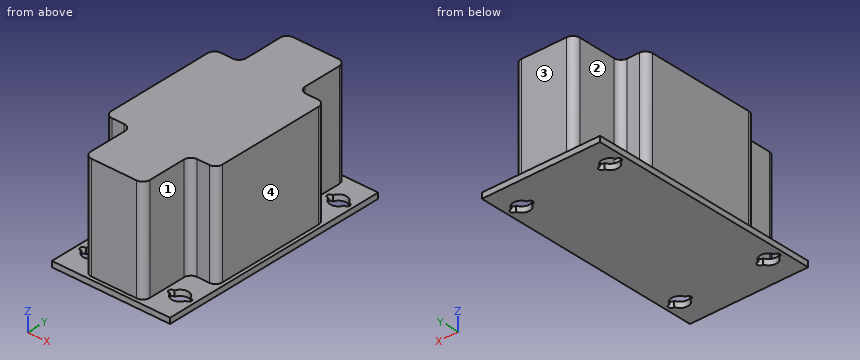
Autodesk Inventor part; units mm, degrees
ref_plane "YZ Plane" through (0, 0, 0) normal (1, 0, 0) x (0, 1, 0)
ref_plane "XZ Plane" through (0, 0, 0) normal (0, 1, 0) x (-1, 0, 0)
ref_plane "XY Plane" through (0, 0, 0) normal (0, 0, 1) x (1, 0, 0)
sketch "Sketch1" plane through (0, 0, 0) normal (0, 0, 1) x (1, 0, 0)
  line L0 (17, 33.5) -> (-17, 33.5)
  line L1 (-17, 33.5) -> (-17, -33.5)
  line L2 (-17, -33.5) -> (17, -33.5)
  line L3 (17, -33.5) -> (17, 33.5)
  line L4 (17, 33.5) -> (-17, -33.5) construction
  line L5 (-17, 33.5) -> (17, -33.5) construction
  line L6 (-12.75, 25.5) -> (12.75, 25.5) construction
  line L7 (12.75, 25.5) -> (12.75, -25.5) construction
  line L8 (12.75, -25.5) -> (-12.75, -25.5) construction
  line L9 (-12.75, -25.5) -> (-12.75, 25.5) construction
  line L10 (-12.75, 25.5) -> (12.75, -25.5) construction
  line L11 (12.75, 25.5) -> (-12.75, -25.5) construction
  line L12 (17, 0) -> (-17, 0) construction
  line L13 (0, 33.5) -> (0, -33.5) construction
  circle A0 centre (12.75, 25.5) radius 2.4
  circle A1 centre (-12.75, 25.5) radius 2.4
  circle A2 centre (12.75, -25.5) radius 2.4
  circle A3 centre (-12.75, -25.5) radius 2.4
  line L14 (12.75, 32.5) -> (12.75, 18.5) construction
  line L15 (16, 17.5) -> (-16, 17.5)
  line L16 (-16, 17.5) -> (-16, -17.5)
  line L17 (-16, -17.5) -> (16, -17.5)
  line L18 (16, -17.5) -> (16, 17.5)
  line L19 (16, 17.5) -> (-16, -17.5) construction
  line L20 (-16, 17.5) -> (16, -17.5) construction
  line L21 (8.5, 17.5) -> (8.5, 32.5)
  line L22 (8.5, 32.5) -> (-8.5, 32.5)
  line L23 (-8.5, 32.5) -> (-8.5, 17.5)
  line L24 (8.5, -17.5) -> (8.5, -32.5)
  line L25 (8.5, -32.5) -> (-8.5, -32.5)
  line L26 (-8.5, -32.5) -> (-8.5, -17.5)
  arc A4 (10.4605, 26.2199) -> (10.4605, 24.7801) centre (10.25, 25.5) ccw
  arc A5 (15.0395, 24.7801) -> (15.0395, 26.2199) centre (15.25, 25.5) ccw
  arc A6 (10.4605, -24.7801) -> (10.4605, -26.2199) centre (10.25, -25.5) ccw
  arc A7 (15.0395, -26.2199) -> (15.0395, -24.7801) centre (15.25, -25.5) ccw
  arc A8 (-10.4605, 24.7801) -> (-10.4605, 26.2199) centre (-10.25, 25.5) ccw
  arc A9 (-15.0395, 26.2199) -> (-15.0395, 24.7801) centre (-15.25, 25.5) ccw
  arc A10 (-10.4605, -26.2199) -> (-10.4605, -24.7801) centre (-10.25, -25.5) ccw
  arc A11 (-15.0395, -24.7801) -> (-15.0395, -26.2199) centre (-15.25, -25.5) ccw
  point P0 (0, 0)
  point P1 (8.5, -17.5)
  point P2 (-8.5, -17.5)
  point P3 (16, 25.5)
  point P4 (9.5, 25.5)
  point P5 (15.0395, 26.2199)
  point P6 (15.0395, 24.7801)
  point P7 (15.0395, -24.7801)
  point P8 (15.0395, -26.2199)
  point P9 (10.4605, -26.2199)
  point P10 (10.4605, -24.7801)
  point P11 (-15.0395, -26.2199)
  point P12 (-15.0395, -24.7801)
  point P13 (-10.4605, -24.7801)
  point P14 (-10.4605, -26.2199)
  point P15 (-15.0395, 24.7801)
  point P16 (-15.0395, 26.2199)
  point P17 (-10.4605, 26.2199)
  point P18 (-10.4605, 24.7801)
  dimension "d0" = 34
  dimension "d1" = 67
  dimension "d19" = 4.8
  dimension "d33" = 51
  dimension "d34" = 25.5
  dimension "d38" = 1
  dimension "d43" = 1
  dimension "d44" = 1
  dimension "d46" = 6.5
  dimension "d47" = 1.5
  dimension "d48" = 1
  dimension "d50" = 16
extrude "Extrusion1" add sketch "Sketch1" along normal blind 1.6 contours L3 L2 L1 L0 | L18 L17 L16 L15 | L15 L23 L22 L21 | L24 L25 L26 L17
extrude "Extrusion2" add sketch "Sketch1" along normal blind 31.6 contours L18 L17 L16 L15 | L15 L23 L22 L21 | L24 L25 L26 L17
fillet "Fillet1" radius 2 12 edges at (16, -17.5, 16.6) (16, 17.5, 16.6) (-16, -17.5, 16.6) (-16, 17.5, 16.6) (8.5, 17.5, 16.6) (8.5, -17.5, 16.6) (8.5, -32.5, 16.6) (-8.5, -32.5, 16.6) (-8.5, -17.5, 16.6) (-8.5, 17.5, 16.6) (-8.5, 32.5, 16.6) (8.5, 32.5, 16.6)
properties part number "SUSTAINA-POWER-DISTRIBUTION-BOARD" material "Acetal Resin, Black"
The listing builds one solid part. Answer for the finished solid, in the listing's coordinates (mm). Face numbers are marked on the shaded views. A direction names the side the tool comes from. Give positions to 0.01 mm unless a question says otherwise; leave off trailing zeros. Order: outer loops, then holes, each group sorted by start corner. A loop starts at its lowest first (then second) coordinate and runs counter-clockwise, first axis right, second up. Notation, with made-up numbers: M 50.5,37.5 L 61.5,37.5 A10 cw 61.5,53.5 Z; hole C 46.5,5 d11. An arc over 180 degrees is marked long. Put each result on its own line as item: value. Start each with the question number.
Item 1: The part is cut by section A-A, the plane x = 4. Determine the outline of the cut face in (y, z), and give its area (3 significant figures).
Item 2: Find the intervals of material crossed by line 1 along Y through (x, z) = (15.25, 1.05); line 2 along Y through (x, z) = (-13.5, 1); line 3 along X through (y, z) = (-0.5, 11), in increasing order.
Item 3: The part is cut by section D-D, the plane y = 9. Determine the outline of the cut face in (x, z), and give its area (3 significant figures).
Item 4: The part is cut by section B-B, the plane x = 13. Determine the outline of the cut face in (y, z), and give its area (3 significant figures).
Item 5: The part is cut by section C-C, the plane z = 20. Determine the outline of the cut face in (x, y), and give its area (3 significant figures).
Item 6: Flat-ended cylindrical pins translate along their axes: P1, Ø1, axis at x = -12, z = 17.5, coming from the +Y side; P2, Ø1, axis at x = -9.5, z = 21, coming from the -Y side; P3, Ø1.4, axis at x = -15.25, y = -25.5, coming from the +Z side (3 decimals); P4, Ø9, axis at y = 23.5, z = 24, coming from the -X side. Find the tip coordinate at first contact, or state that the pin passes through.
Item 7: Which of the six approach directions +Z, -Z, +X, -X, +Y, -Y give full straight-line access (tool end or side, diameter ignored) to the marked faces 1, 2, 3 and 4?
Answer key:
1. outline: M -33.5,0 L 33.5,0 L 33.5,1.6 L 32.5,1.6 L 32.5,31.6 L -32.5,31.6 L -32.5,1.6 L -33.5,1.6 Z
1. area: 2,060 mm²
2. line 1: y = -33.5 to -26.25, -24.75 to 24.75, 26.25 to 33.5
2. line 2: y = -33.5 to -27.78, -23.22 to 23.22, 27.78 to 33.5
2. line 3: x = -16 to 16
3. outline: M -17,0 L 17,0 L 17,1.6 L 16,1.6 L 16,31.6 L -16,31.6 L -16,1.6 L -17,1.6 Z
3. area: 1,010 mm²
4. outline: M -33.5,0 L -27.89,0 L -27.89,1.6 L -33.5,1.6 Z; M -23.11,0 L 23.11,0 L 23.11,1.6 L 17.5,1.6 L 17.5,31.6 L -17.5,31.6 L -17.5,1.6 L -23.11,1.6 Z; M 27.89,0 L 33.5,0 L 33.5,1.6 L 27.89,1.6 Z
4. area: 1,140 mm²
5. outline: M -16,-15.5 A2 ccw -14,-17.5 L -10.5,-17.5 A2 cw -8.5,-19.5 L -8.5,-30.5 A2 ccw -6.5,-32.5 L 6.5,-32.5 A2 ccw 8.5,-30.5 L 8.5,-19.5 A2 cw 10.5,-17.5 L 14,-17.5 A2 ccw 16,-15.5 L 16,15.5 A2 ccw 14,17.5 L 10.5,17.5 A2 cw 8.5,19.5 L 8.5,30.5 A2 ccw 6.5,32.5 L -6.5,32.5 A2 ccw -8.5,30.5 L -8.5,19.5 A2 cw -10.5,17.5 L -14,17.5 A2 ccw -16,15.5 Z
5. area: 1,630 mm²
6. P1: stops at y = 17.5
6. P2: stops at y = -18.18
6. P3: passes through
6. P4: stops at x = -8.56
7. face 1: +Z, +X, -Y
7. face 2: +Z, -X, +Y
7. face 3: +Z, +X, -X, +Y
7. face 4: +Z, +X, +Y, -Y
